```python
from build123d import *

# Parameters (mm, degrees)
BASPROSKE_W         = 3
BASPROSKE_H         = 16.5
TOOTHCUT_DEPTH      = 24.526580712
TEETHCUTS_COUNT     = 20
TEETHCUTS_ANGLE     = 342
SKETCH_3_R          = 2.5
CUT_EXTRUDE_2_DEPTH = 10
SKETCH_4_R          = 10
EXTRUDE_4_DEPTH     = 3.4
SKETCH_6_R          = 2.5
CUT_EXTRUDE_3_DEPTH = 24.997285258
SKETCH_2_R          = 1.25
EXTRUDE_5_DEPTH     = 3
SKETCH_7_R          = 2.5
CUT_EXTRUDE_4_DEPTH = 43.823439076
EXTRUDE_6_DEPTH     = 3
EXTRUDE_START       = -3
EXTRUDE_14_DEPTH    = 3


with BuildPart() as part:
    # BasProSke → Base-Revolve (revolve)
    with BuildSketch(Plane(origin=(0, 0, 0), x_dir=(1, 0, 0), z_dir=(0, 1, 0)), mode=Mode.PRIVATE) as base_revolve_sk:
        with Locations((1.5, 8.25)):
            Rectangle(BASPROSKE_W, BASPROSKE_H)
    revolve(base_revolve_sk.sketch.rotate(Axis((-10, 0, 0), (1, 0, 0)), 180), axis=Axis((-10, 0, 0), (1, 0, 0)))

    # TooCutSke → ToothCut (cut, through all)
    with BuildSketch(Plane(origin=(0, 0, 0), x_dir=(0, 0, -1), z_dir=(1, 0, 0))):
        with BuildLine():
            ThreePointArc((0.74381438, 13.102904875), (0, 13.124), (-0.74381438, 13.102904875))
            ThreePointArc((-0.74381438, 13.102904875), (-1.226473103, 14.852072512), (-2.209965745, 16.376962373))
            ThreePointArc((-2.209965745, 16.376962373), (0, 16.5254), (2.209965745, 16.376962373))
            ThreePointArc((2.209965745, 16.376962373), (1.226473103, 14.852072512), (0.74381438, 13.102904875))
        make_face()
    toothcut = extrude(amount=TOOTHCUT_DEPTH, mode=Mode.SUBTRACT)

    # TeethCuts: ToothCut ×20 about axis
    teethcuts_axis = Axis((-10, 0, 0), (1, 0, 0))
    for i in range(1, TEETHCUTS_COUNT):
        add(toothcut.rotate(teethcuts_axis, i * TEETHCUTS_ANGLE / (TEETHCUTS_COUNT - 1)), mode=Mode.SUBTRACT)

    # 草图3 → 切除-拉伸2 (cut)
    with BuildSketch(Plane.ZY):
        Circle(SKETCH_3_R)
        with Locations((0, 27)):
            Circle(SKETCH_3_R)
    extrude(amount=-CUT_EXTRUDE_2_DEPTH, mode=Mode.SUBTRACT)

    # 草图4 → 凸台-拉伸4 (add)
    with BuildSketch(Plane.ZY):
        with Locations(Location((0, 0, 0), (0, 0, 180))):
            Circle(SKETCH_4_R)
    extrude(amount=EXTRUDE_4_DEPTH)

    # 草图6 → 切除-拉伸3 (cut, through all)
    with BuildSketch(Plane.ZY.offset(3.4)):
        Circle(SKETCH_6_R)
    extrude(amount=-CUT_EXTRUDE_3_DEPTH, mode=Mode.SUBTRACT)

    # 草图2 → 凸台-拉伸5 (add)
    with BuildSketch(Plane.ZY):
        with BuildLine():
            Line((-3.456909192, -0.547520628), (-9.088549934, 35.009259634))
            ThreePointArc((-9.088549934, 35.009259634), (-6.179161369, 39.013689454), (-2.174731549, 36.104300889))
            Line((-2.174731549, 36.104300889), (3.456909192, 0.547520628))
            ThreePointArc((3.456909192, 0.547520628), (0.547520628, -3.456909192), (-3.456909192, -0.547520628))
        make_face()
        with Locations((-4.067296091, 25.679896855)):
            Circle(SKETCH_2_R, mode=Mode.SUBTRACT)
        with Locations((-5.631640741, 35.556780261)):
            Circle(SKETCH_2_R, mode=Mode.SUBTRACT)
    extrude(amount=-EXTRUDE_5_DEPTH)

    # 草图7 → 切除-拉伸4 (cut, through all)
    with BuildSketch(Plane(origin=(3, 0, 0), x_dir=(0, 0, -1), z_dir=(1, 0, 0))):
        with Locations(Location((0, 0, 0), (0, 0, 180))):
            Circle(SKETCH_7_R)
    extrude(amount=-CUT_EXTRUDE_4_DEPTH, mode=Mode.SUBTRACT)

    # 草图8 → 凸台-拉伸6 (add)
    with BuildSketch(Plane.ZY):
        Polygon((-7.841095822, 14.51782409), (-7.136285925, 14.87694267), (-5.713237213, 13.698373831), (-9.125006953, 35.341391045), align=None)
    extrude(amount=-EXTRUDE_6_DEPTH)

    # 草图9 → 凸台-拉伸14 (add)
    with BuildSketch(Plane.ZY.offset(EXTRUDE_START)):
        with BuildLine():
            Line((2.971070911, 16.230303067), (-2.174731549, 36.104300889))
            Line((-2.174731549, 36.104300889), (1.200581171, 14.793415086))
            Line((1.200581171, 14.793415086), (1.303832307, 15.021332463))
            Line((1.303832307, 15.021332463), (1.648552458, 15.68967923))
            Line((1.648552458, 15.68967923), (2.189783121, 16.354046896))
            ThreePointArc((2.189783121, 16.354046896), (2.581168673, 16.29685762), (2.971070911, 16.230303067))
        make_face()
    extrude(amount=EXTRUDE_14_DEPTH)


solid = part.part
```
Verification items for the finished model (mm, model axes). A direction names the side the tool comes from. Coordinates: 2 decimals unless noted, no trailing zeros. Loops run counter-clockwise (first coordinate to the right, second up) from the corner with the lowest first, then second, coordinate; pieces in that order, holes last. Notation, with made-up numbers: (25, 18.25) -> (31, 18.25) arc R32 cw to (31, 54.25) -> close; hole circle Ø4 at (17.5, -25.75). An arc over 180 degrees is marked (long way). Answer in a Markdown table with one row per item. Add a question column.
1. Section check A-A, the plane y = 0. Enter the section's corners in (x, z), then the cut area to 3 significant figures.
2. Access from +Z, -Z, +X, -X, +Y, -Y to the whole of each face (thin tool, end or side, straight path). Record for faces 1 (the face through (1, 6, -14)), 2 (the face through (1.48, 12.7, -7.73)), 3 (the face through (1, 6, 14)).
3. Depth check by flat-ended pin: P1, Ø10, axis at y = 22.5, z = -7, coming from the -X side; P2, Ø1.5, axis at y = 35.56, z = -5.63, coming from the +X side; P3, Ø1, axis at x = -2, z = -9, coming from the -Y side. Enter the tip coordinate at first touch or a pass-through.
4. Section check B-B, the plane z = 0. Enter the section's corners in (x, y).
5. Draft check along Y on faces 4 (the face through (1.479, -14.464, 3.427)), 5 (the face through (1.521, 26.028, 0.434)), 6 (the face through (0, 11, -1)), 7 (the face through (1.48, -11.3, 9.73)). Enter one of: +Y half, -Y half, draft (parallel to the pull), parting line (faces both ways), or undercut.
6. Material ranges on probe 1 along Z at (x, y) = (0.5, 0); probe 2 along Y at (x, z) = (1.25, -11.5); probe 3 along Y at (x, z) = (-1, 0), recorded low to high. Write a range as [from, to].
7. Section check C-C, the plane x = -2.25. Enter the section's corners in (y, z).
8. Section check D-D, the plane y = 6.5. Enter the section's corners in (x, z).
Derived:
| question | item | result |
|---|---|---|
| 1 | outline | (-3.4, -10) -> (0, -10) -> (0, -13.12) -> (3, -13.12) -> (3, -2.5) -> (-3.4, -2.5) -> close; (-3.4, 2.5) -> (3, 2.5) -> (3, 13.12) -> (0, 13.12) -> (0, 10) -> (-3.4, 10) -> close |
| 1 | area | 115 mm² |
| 2 | face 1 | -Z, +X, -X |
| 2 | face 2 | +X, -X |
| 2 | face 3 | +Z, +X, -X |
| 3 | P1 | stops at x = 0 |
| 3 | P2 | passes through |
| 3 | P3 | stops at y = -5.27 |
| 4 | outline | (-3.4, -10) -> (0, -10) -> (0, -13.12) -> (3, -13.12) -> (3, -2.5) -> (-3.4, -2.5) -> close; (-3.4, 2.5) -> (3, 2.5) -> (3, 27.71) -> (0, 27.71) -> (0, 10) -> (-3.4, 10) -> close |
| 5 | face 4 | undercut |
| 5 | face 5 | +Y half |
| 5 | face 6 | draft |
| 5 | face 7 | -Y half |
| 6 | probe 1 | z = [-13.12, -2.5], [2.5, 13.12] |
| 6 | probe 2 | y = [-11.83, -10.11], [-7.33, 7.33], [10.11, 11.83] |
| 6 | probe 3 | y = [-10, -2.5], [2.5, 10] |
| 7 | outline | circle Ø20 at (0, 0); hole circle Ø5 at (0, 0) |
| 8 | outline | (-3.4, -7.6) -> (0, -7.6) -> (0, -14.44) -> (3, -14.44) -> (3, 14.44) -> (0, 14.44) -> (0, 7.6) -> (-3.4, 7.6) -> close |
